Geometry check sheet. Reference: the model listing, model coordinates, mm. Face numbers are marked on the shaded views. Give positions to 0.01 mm unless a question says otherwise; leave off trailing zeros. Loops run counter-clockwise (first coordinate to the right, second up) from the corner with the lowest first, then second, coordinate; pieces in that order, holes last.
1. Cross-section at B-B, the plane x = -25. Record the cut outline in (y, z).
2. Go/stop test with flat-tipped pins: pin 1 Ø1 at (x, z) = (-26.5, 25.5) entering from -Y; pin 2 Ø3 at (x, z) = (4.5, 28.5) entering from +Y; pin 3 Ø0.6 at (x, z) = (12, 0.5) entering from -Y; pin 4 Ø1.8 at (x, y) = (25, 14.43) entering from +Z. Record where each tip stops, or that it passes through.
3. Cross-section at A-A, the plane y = 5. Record the cut outline in (x, z), plus the area to 3 significant figures.
4. Material ranges on L1, parallel to X at y = 10, z = 41.5; L2, parallel to Y at x = 37, z = 47.5; L3, parallel to Y at x = 25, z = 1, recorded low to high.
5. Release check for a two-part mould opening along Y. For the marked faces 1 and 2 record: +Y half, -Y half, draft (parallel to the pull), parting line (faces both ways), or undercut.
6. Cross-section at C-C, the plane z = 7. Record the cut outline in (x, y).
7. Cross-section at D-D, the plane y = 34.5. Record the cut outline in (x, z).
from build123d import *

# Parameters (mm, degrees)
F0_R     = 1.5
F0_W     = 10
F0_H     = 5
F0_W_2   = 17.5
F0_W_3   = 5
F1_DEPTH = 2
F3_DEPTH = 60


with BuildPart() as f1:
    # F0 (on Top) → F1 (new body)
    with BuildSketch(Plane.XY):
        Polygon((0, -46.1880215352), (2.5, -44.7446458622), (-2.5, -44.7446458622), align=None)
        Polygon((-2.5, 44.7446458622), (2.5, 44.7446458622), (0, 46.1880215352), align=None)
        Polygon((-2.5, -44.7446458622), (2.5, -44.7446458622), (2.5, -42.4352447854), (0, -43.8786204584), (-2.5, -42.4352447854), align=None)
        Polygon((2.5, 42.4352447854), (2.5, 44.7446458622), (-2.5, 44.7446458622), (-2.5, 42.4352447854), (0, 43.8786204584), align=None)
        Polygon((40, -23.0940107676), (40, 23.0940107676), (2.5, 44.7446458622), (2.5, 42.4352447854), (38, 21.9393102292), (38, 2.5), (38, 2), (38, -2), (38, -2.5), (38, -21.9393102292), (2.5, -42.4352447854), (2.5, -44.7446458622), align=None)
        Polygon((-2.5, 42.4352447854), (-2.5, 44.7446458622), (-40, 23.0940107676), (-40, -23.0940107676), (-2.5, -44.7446458622), (-2.5, -42.4352447854), (-38, -21.9393102292), (-38, -2.5), (-38, -2), (-38, 2), (-38, 2.5), (-38, 21.9393102292), align=None)
        Polygon((-2.5, 21.6506350946), (-2.5, 33.1976404784), (-30, 17.3205080757), (-30, 2.5), (-20, 2.5), (-20, 11.5470053838), align=None)
        with Locations((-25, 14.4337567297)):
            Circle(F0_R, mode=Mode.SUBTRACT)
        Polygon((30, 17.3205080757), (2.5, 33.1976404784), (2.5, 21.6506350946), (20, 11.5470053838), (20, 2.5), (30, 2.5), align=None)
        with Locations((25, 14.4337567297)):
            Circle(F0_R, mode=Mode.SUBTRACT)
        Polygon((2.5, 21.6506350946), (2.5, 33.1976404784), (0, 34.6410161514), (-2.5, 33.1976404784), (-2.5, 21.6506350946), (0, 23.0940107676), align=None)
        Polygon((2.5, 33.1976404784), (2.5, 42.4352447854), (0, 43.8786204584), (-2.5, 42.4352447854), (-2.5, 33.1976404784), (0, 34.6410161514), align=None)
        Polygon((-30, -17.3205080757), (-2.5, -33.1976404784), (-2.5, -21.6506350946), (-20, -11.5470053838), (-20, -2.5), (-30, -2.5), align=None)
        with Locations((-25, -14.4337567297)):
            Circle(F0_R, mode=Mode.SUBTRACT)
        Polygon((0, -34.6410161514), (2.5, -33.1976404784), (2.5, -21.6506350946), (0, -23.0940107676), (-2.5, -21.6506350946), (-2.5, -33.1976404784), align=None)
        Polygon((2.5, -21.6506350946), (2.5, -33.1976404784), (30, -17.3205080757), (30, -2.5), (20, -2.5), (20, -11.5470053838), align=None)
        with Locations((25, -14.4337567297)):
            Circle(F0_R, mode=Mode.SUBTRACT)
        with Locations((25, 0)):
            Rectangle(F0_W, F0_H)
        with BuildLine():
            Line((38, 2), (38, 2.5))
            Line((38, 2.5), (30, 2.5))
            Line((30, 2.5), (30, -2.5))
            Line((30, -2.5), (38, -2.5))
            Line((38, -2.5), (38, -2))
            ThreePointArc((38, -2), (36, 0), (38, 2))
        make_face()
        with Locations((11.25, 0)):
            Rectangle(F0_W_2, F0_H)
        Polygon((2.5, 2.5), (2.5, 21.6506350946), (0, 23.0940107676), (-2.5, 21.6506350946), (-2.5, 2.5), align=None)
        with Locations((-11.25, 0)):
            Rectangle(F0_W_2, F0_H)
        with Locations((-25, 0)):
            Rectangle(F0_W, F0_H)
        with BuildLine():
            Line((-30, 2.5), (-38, 2.5))
            Line((-38, 2.5), (-38, 2))
            ThreePointArc((-38, 2), (-36, 0), (-38, -2))
            Line((-38, -2), (-38, -2.5))
            Line((-38, -2.5), (-30, -2.5))
            Line((-30, -2.5), (-30, 2.5))
        make_face()
        Polygon((0, -23.0940107676), (2.5, -21.6506350946), (2.5, -2.5), (-2.5, -2.5), (-2.5, -21.6506350946), align=None)
        Rectangle(F0_W_3, F0_H)
        Polygon((0, -43.8786204584), (2.5, -42.4352447854), (2.5, -33.1976404784), (0, -34.6410161514), (-2.5, -33.1976404784), (-2.5, -42.4352447854), align=None)
        with BuildLine():
            ThreePointArc((-38, -2), (-36, 0), (-38, 2))
            Line((-38, 2), (-38, -2))
        make_face()
        with BuildLine():
            Line((38, -2), (38, 2))
            ThreePointArc((38, 2), (36, 0), (38, -2))
        make_face()
    extrude(amount=F1_DEPTH)

    # F2 (on face) → F3 (join)
    with BuildSketch(Plane.XY.offset(2)):
        Polygon((-40, 23.0940107676), (-40, -23.0940107676), (0, -46.1880215352), (40, -23.0940107676), (40, 23.0940107676), (0, 46.1880215352), align=None)
        Polygon((0, -43.8786204584), (-38, -21.9393102292), (-38, -2), (-38, 2), (-38, 21.9393102292), (0, 43.8786204584), (38, 21.9393102292), (38, 2), (38, -2), (38, -21.9393102292), align=None, mode=Mode.SUBTRACT)
        with BuildLine():
            Line((-38, 2), (-38, -2))
            ThreePointArc((-38, -2), (-36, 0), (-38, 2))
        make_face()
        with BuildLine():
            ThreePointArc((38, 2), (36, 0), (38, -2))
            Line((38, -2), (38, 2))
        make_face()
    extrude(amount=F3_DEPTH)


solid = f1.part
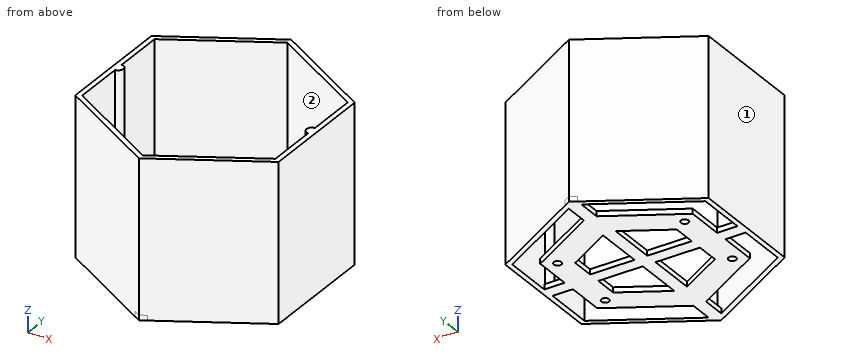
Result:
1. outline: (-31.75, 0) - (-29.44, 0) - (-29.44, 62) - (-31.75, 62) - close; (-20.21, 0) - (-15.93, 0) - (-15.93, 2) - (-20.21, 2) - close; (-12.93, 0) - (12.93, 0) - (12.93, 2) - (-12.93, 2) - close; (15.93, 0) - (20.21, 0) - (20.21, 2) - (15.93, 2) - close; (29.44, 0) - (31.75, 0) - (31.75, 62) - (29.44, 62) - close
2. pin 1: stops at y = -31.18
2. pin 2: stops at y = 44.46
2. pin 3: stops at y = -39.43
2. pin 4: passes through
3. outline: (-40, 0) - (-38, 0) - (-38, 62) - (-40, 62) - close; (-30, 0) - (-20, 0) - (-20, 2) - (-30, 2) - close; (-2.5, 0) - (2.5, 0) - (2.5, 2) - (-2.5, 2) - close; (20, 0) - (30, 0) - (30, 2) - (20, 2) - close; (38, 0) - (40, 0) - (40, 62) - (38, 62) - close
3. area: 298 mm2
4. L1: x = -40 to -38, 38 to 40
4. L2: y = -24.83 to -22.52, -1.73 to 1.73, 22.52 to 24.83
4. L3: y = -31.75 to -29.44, -20.21 to -15.93, -12.93 to 12.93, 15.93 to 20.21, 29.44 to 31.75
5. face 1: draft
5. face 2: undercut
6. outline: (-40, -23.09) - (0, -46.19) - (40, -23.09) - (40, 23.09) - (0, 46.19) - (-40, 23.09) - close; hole (-38, -21.94) - (0, -43.88) - (38, -21.94) - (38, -2) arc R2 cw to (38, 2) - (38, 21.94) - (0, 43.88) - (-38, 21.94) - (-38, 2) arc R2 cw to (-38, -2) - close
7. outline: (-20.24, 0) - (-16.24, 0) - (-16.24, 62) - (-20.24, 62) - close; (-2.5, 0) - (2.5, 0) - (2.5, 2) - (-2.5, 2) - close; (16.24, 0) - (20.24, 0) - (20.24, 62) - (16.24, 62) - close
